```python
from build123d import *

# Parameters (mm, degrees)
F1_DEPTH = 20
F2_R     = 5.5
F2_R_2   = 4
F2_R_3   = 1.395
F3_DEPTH = 2
F4_DEPTH = 112.584302492
F6_DEPTH = 10.001
F8_DEPTH = 5.5


with BuildPart() as f1:
    # F0 (on Front) → F1 (new body)
    with BuildSketch(Plane.XZ):
        with BuildLine():
            Line((30, 51.9615242271), (0, 0))
            Line((0, 0), (130, 0))
            Line((130, 0), (130, 10))
            Line((130, 10), (88.0384757729, 10))
            ThreePointArc((88.0384757729, 10), (82.8620948709, 10.6814834742), (78.0384757729, 12.6794919243))
            Line((78.0384757729, 12.6794919243), (62.2390923627, 21.8012701892))
            ThreePointArc((62.2390923627, 21.8012701892), (61.5402036233, 22.7120797272), (61.6900542571, 23.8503082949))
            Line((61.6900542571, 23.8503082949), (62.9400542571, 26.0153718044))
            Line((62.9400542571, 26.0153718044), (45.6195461814, 36.0153718044))
            Line((45.6195461814, 36.0153718044), (44.3695461814, 33.8503082949))
            ThreePointArc((44.3695461814, 33.8503082949), (43.4587366433, 33.1514195555), (42.3205080757, 33.3012701892))
            Line((42.3205080757, 33.3012701892), (27.5980762114, 41.8012701892))
            ThreePointArc((27.5980762114, 41.8012701892), (26.8991874719, 42.7120797272), (27.0490381057, 43.8503082949))
            Line((27.0490381057, 43.8503082949), (31.2990381057, 51.2115242271))
            Line((31.2990381057, 51.2115242271), (30, 51.9615242271))
        make_face()
        with BuildLine():
            ThreePointArc((13.0711054025, 8.6635187293), (10.3758012826, 11.6884456075), (10.8062850623, 15.7170347689))
            Line((10.8062850623, 15.7170347689), (23.0490381057, 36.9221050646))
            ThreePointArc((23.0490381057, 36.9221050646), (26.0850698991, 39.2517341961), (29.8791651246, 38.7522320835))
            Line((29.8791651246, 38.7522320835), (78.2416697508, 10.8301270189))
            ThreePointArc((78.2416697508, 10.8301270189), (80.5712988822, 5.2059047745), (75.7416697508, 1.5))
            Line((75.7416697508, 1.5), (28.8649813291, 1.5))
            Line((28.8649813291, 1.5), (13.0711054025, 8.6635187293))
        make_face(mode=Mode.SUBTRACT)
    extrude(amount=F1_DEPTH)

    # F2 (on face) → F3 (cut)
    with BuildSketch(Plane(origin=(0, 0, 0), x_dir=(0, -1, 0), z_dir=(-0.8660254038, 0, 0.5))):
        with Locations((10, 7.5)):
            Circle(F2_R)
        with Locations((10, 7.5)):
            Circle(F2_R_2, mode=Mode.SUBTRACT)
        with Locations((5, 25)):
            Circle(F2_R_3)
        with Locations((15, 25)):
            Circle(F2_R_3)
        with Locations((15, 32)):
            Circle(F2_R_3)
        with Locations((15, 39)):
            Circle(F2_R_3)
        with Locations((5, 39)):
            Circle(F2_R_3)
        with Locations((5, 32)):
            Circle(F2_R_3)
    extrude(amount=-F3_DEPTH, mode=Mode.SUBTRACT)

    # F4 (cut, through all): a face of the model
    f4_faces = [f1.faces().sort_by_distance(p)[0] for p in [
        (3.75, -10, 6.4951905284),
    ]]
    extrude(f4_faces, amount=-F4_DEPTH, mode=Mode.SUBTRACT)

    # F5 (on face) → F6 (cut, through all)
    with BuildSketch(Plane.XY.offset(10)):
        with BuildLine():
            Line((130, -13), (130, -10))
            Line((130, -10), (130, -7))
            Line((130, -7), (113, -7))
            ThreePointArc((113, -7), (110.8786796564, -7.8786796564), (110, -10))
            ThreePointArc((110, -10), (110.8786796564, -12.1213203436), (113, -13))
            Line((113, -13), (130, -13))
        make_face()
        with BuildLine():
            Line((130, -20), (130, -15))
            Line((130, -15), (98, -15))
            ThreePointArc((98, -15), (95.8786796564, -15.8786796564), (95, -18))
            Line((95, -18), (95, -20))
            Line((95, -20), (130, -20))
        make_face()
        with BuildLine():
            Line((98, -5), (130, -5))
            Line((130, -5), (130, 0))
            Line((130, 0), (95, 0))
            Line((95, 0), (95, -2))
            ThreePointArc((95, -2), (95.8786796564, -4.1213203436), (98, -5))
        make_face()
    extrude(amount=-F6_DEPTH, mode=Mode.SUBTRACT)

    # F7 (on face) → F8 (cut, through all)
    with BuildSketch(Plane(origin=(27, 0, 46.7653718044), x_dir=(0.8660254038, 0, -0.5), z_dir=(0.5, 0, 0.8660254038))):
        with BuildLine():
            Line((35, -6), (28, -6))
            ThreePointArc((28, -6), (25.1715728753, -7.1715728753), (24, -10))
            ThreePointArc((24, -10), (25.1715728753, -12.8284271247), (28, -14))
            Line((28, -14), (35, -14))
            ThreePointArc((35, -14), (37.8284271247, -12.8284271247), (39, -10))
            ThreePointArc((39, -10), (37.8284271247, -7.1715728753), (35, -6))
        make_face()
    extrude(amount=-F8_DEPTH, mode=Mode.SUBTRACT)


solid = f1.part
```
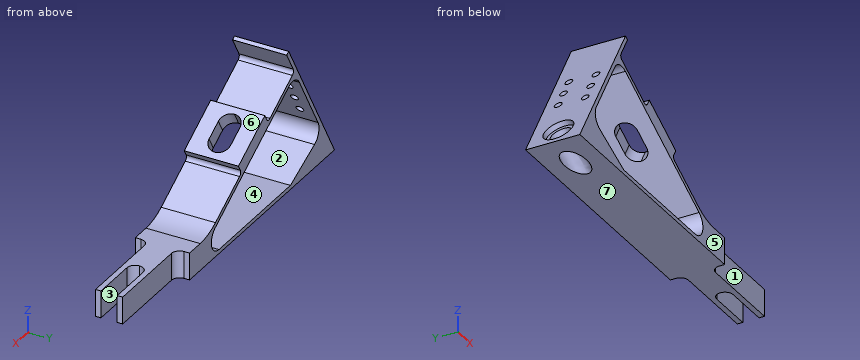
Read the model definition and answer for the solid it produces. Units are mm, in the model's axes. Face numbers are marked on the shaded views. A direction names the side the tool comes from. Coordinates: 2 decimals unless noted, no trailing zeros. Write each loop counter-clockwise with the first axis right and the second up, starting at its lowest first coordinate (ties: lowest second). Pieces come first, ordered by that corner, then holes. Notation, with made-up numbers: (19.5, 14) -> (68.5, 14) arc R24 cw to (68.5, 43) -> close; hole circle Ø6 at (-31, 30.25). An arc over 180 degrees is marked (long way). Return JSON: item names as keys, results as strings.
1. A cutting plane is placed at B-B (z = 18.5). Determine the outline of the cut face in (x, y).
Found:
{"outline": "(10.68, -20) -> (12.41, -20) -> (12.41, 0) -> (10.68, 0) -> close; (64.96, -20) -> (67.96, -20) -> (67.96, 0) -> (64.96, 0) -> close"}
2. A cutting plane is placed at C-C (x = 103.5). Determine the outline of the cut face in (y, z).
Found:
{"outline": "(-15, 0) -> (-5, 0) -> (-5, 10) -> (-15, 10) -> close"}
3. Each of these flat-tipped pins is pushed along its axis until it touches: P1, Ø1.6, axis at y = -18.5, z = 6, coming from the +X side; P2, Ø12, axis at x = 60.5, z = 38.5, coming from the +Y side; P3, Ø3, axis at x = 123, z = 7, coming from the +Y side; P4, Ø1.5, axis at y = -11.5, z = 23.5, coming from the -X side. Where does it stop, or does it pass through?
Found:
{"P1": "x = 95.02", "P2": "through", "P3": "y = -5", "P4": "x = 13.13"}
4. A cutting plane is placed at D-D (x = 90). Determine the outline of the cut face in (y, z).
Found:
{"outline": "(-20, 0) -> (0, 0) -> (0, 10) -> (-20, 10) -> close"}
5. A cutting plane is placed at A-A (x = 39). Determine the outline of the cut face in (y, z).
Found:
{"outline": "(-20, 0) -> (0, 0) -> (0, 1.5) -> (-20, 1.5) -> close; (-20, 33.49) -> (0, 33.49) -> (0, 35.22) -> (-20, 35.22) -> close"}
6. Determine the mould class of the marked faces 4, 5, 6 and 7 for opening direction Z: pulls with the +Z half, pulls with the -Z half, needs draft (parallel to the pull), parting line crosses it, or undercut.
Found:
{"face 4": "undercut", "face 5": "needs draft", "face 6": "pulls with the +Z half", "face 7": "pulls with the -Z half"}
7. Find the intervals of material crossed by line 1 along Y through (x, z) = (122, 6); line 2 along X through (y, z) = (-17, 34); line 3 along X through (y, z) = (-10.5, 34.5), in increasing order. Write a range as from..to.
Found:
{"line 1": "-15..-13, -7..-5", "line 2": "19.63..21.36, 38.11..41.11, 44.46..49.11", "line 3": "19.92..21.65, 37.24..40.24, 44.74..47.67"}
8. A tool of negligible diameter and unlimited length cuts with its end or side. For the marked faces 1, 2 and 3, from which of +Z, -Z, +X, -X, +Y, -Y can it reach the whole face along a straight path? Write none if from no direction.
Found:
{"face 1": "+Z, -Z, +X, -Y", "face 2": "+Y, -Y", "face 3": "+Z, -Z, +X"}
